```python
from build123d import *

# Parameters (mm, degrees)
SKETCH1_W           = 50
SKETCH1_H           = 50
SKETCH1_R           = 3.57
SKETCH1_R_2         = 2.51
BOSS_EXTRUDE1_DEPTH = 6.35
SKETCH2_R           = 6
SKETCH2_R_2         = 5.05
CUT_EXTRUDE1_DEPTH  = 1.75
SKETCH3_W           = 5.25
SKETCH3_H           = 6.7
CUT_EXTRUDE2_DEPTH  = 7
SKETCH4_W           = 2.785
SKETCH4_H           = 4.18
SKETCH4_W_2         = 2.79
SKETCH4_H_2         = 4.8
BOSS_EXTRUDE3_DEPTH = 6.7
FILLET1_R           = 6.17


with BuildPart() as part:
    # Sketch1 → Boss-Extrude1 (new body)
    with BuildSketch(Plane.XY):
        Rectangle(SKETCH1_W, SKETCH1_H)
        with Locations((-15, 15)):
            Circle(SKETCH1_R, mode=Mode.SUBTRACT)
        with Locations((15, 15)):
            Circle(SKETCH1_R, mode=Mode.SUBTRACT)
        with Locations((15, -15)):
            Circle(SKETCH1_R_2, mode=Mode.SUBTRACT)
        with Locations((-15, -15)):
            Circle(SKETCH1_R_2, mode=Mode.SUBTRACT)
        with Locations((-10, 0)):
            Circle(SKETCH1_R_2, mode=Mode.SUBTRACT)
        with Locations((0, 10)):
            Circle(SKETCH1_R_2, mode=Mode.SUBTRACT)
        with Locations((10, 0)):
            Circle(SKETCH1_R_2, mode=Mode.SUBTRACT)
        with Locations((0, -10)):
            Circle(SKETCH1_R_2, mode=Mode.SUBTRACT)
        Circle(SKETCH1_R_2, mode=Mode.SUBTRACT)
    extrude(amount=BOSS_EXTRUDE1_DEPTH)

    # Sketch2 → Cut-Extrude1 (cut)
    with BuildSketch(Plane.XY.offset(6.35)):
        with Locations((-15, 15)):
            Circle(SKETCH2_R)
        with Locations((15, 15)):
            Circle(SKETCH2_R)
        with Locations((-15, -15)):
            Circle(SKETCH2_R_2)
        with Locations((15, -15)):
            Circle(SKETCH2_R_2)
    extrude(amount=-CUT_EXTRUDE1_DEPTH, mode=Mode.SUBTRACT)

    # Sketch3 → Cut-Extrude2 (cut)
    with BuildSketch(Plane.XY.offset(6.35)):
        with Locations((-22.375, 0)):
            Rectangle(SKETCH3_W, SKETCH3_H)
        with Locations((22.375, 0)):
            Rectangle(SKETCH3_W, SKETCH3_H)
    extrude(amount=-CUT_EXTRUDE2_DEPTH, mode=Mode.SUBTRACT)

    # Sketch4 → Boss-Extrude3 (add)
    with BuildSketch(Plane.XZ.offset(-3.35)):
        with Locations((-23.6075, 2.09)):
            Rectangle(SKETCH4_W, SKETCH4_H)
        with Locations((23.605, 2.4)):
            Rectangle(SKETCH4_W_2, SKETCH4_H_2)
    extrude(amount=BOSS_EXTRUDE3_DEPTH)

    # Fillet1
    fillet1_edges = [part.edges().sort_by_distance(p)[0] for p in [
        (25, -25, 3.175),
        (-25, -25, 3.175),
        (-25, 25, 3.175),
        (25, 25, 3.175),
    ]]
    fillet(fillet1_edges, radius=FILLET1_R)


solid = part.part
```
Check sheet for the modelled part. Datum: model origin and axes. Units: mm. A direction names the side the tool comes from. Round coordinates to 2 decimals unless told otherwise and drop trailing zeros. Order: outer loops, then holes, each group sorted by start corner. A loop starts at its lowest first (then second) coordinate and runs counter-clockwise, first axis right, second up. Notation, with made-up numbers: (77.5, -13.75) -> (111.5, -13.75) arc R18 ccw to (111.5, 20.25) -> close; hole circle Ø7 at (-21, 71.25). An arc over 180 degrees is marked (long way). Use CSV: the item, a comma, the result in double quotes.
(1) Cross-section at D-D (z = 2). Count the separate pieces of the cut face and the enclosed holes in it, and give its area (3 significant figures).
Worked out:
separate pieces,"1"
enclosed holes,"11"
area,"2,220 mm²"
(2) Cross-section at C-C (y = -15). Record the boundary of the cut face in (x, z).
Worked out:
outline,"(-25, 0) -> (-17.51, 0) -> (-17.51, 4.6) -> (-20.05, 4.6) -> (-20.05, 6.35) -> (-25, 6.35) -> close; (-12.49, 0) -> (12.49, 0) -> (12.49, 4.6) -> (9.95, 4.6) -> (9.95, 6.35) -> (-9.95, 6.35) -> (-9.95, 4.6) -> (-12.49, 4.6) -> close; (17.51, 0) -> (25, 0) -> (25, 6.35) -> (20.05, 6.35) -> (20.05, 4.6) -> (17.51, 4.6) -> close"
(3) Tool access check on faces 1 (the face through (17, -17, 4.6)), 2 (the face through (0, 25, 3)), 3 (the face through (-22.215, 0, 2)), 4 (the face through (24, 0, 4.8)). Record the directions out of +Z, -Z, +X, -X, +Y, -Y that give a thin tool (end or side, any length) a straight path to the whole face; none if there is none.
Worked out:
face 1,"+Z"
face 2,"+Z, -Z, +X, -X, +Y"
face 3,"+Z, -Z"
face 4,"+Z, +X"
(4) Draft check along X on faces 5 (the face through (0, -5, 6.35)), 6 (the face through (-25, 0, 3)), 7 (the face through (-0.33, -7.51, 3.13)). Enter one of: pulls with the +X half, pulls with the -X half, needs draft (parallel to the pull), parting line crosses it, or undercut.
Worked out:
face 5,"needs draft"
face 6,"pulls with the -X half"
face 7,"undercut"
(5) Material ranges on line 1 along Y through (x, z) = (0, 3.5); line 2 along Y through (x, z) = (-15, 5); line 3 along X through (y, z) = (15, 1.1), recorded low to high. Write a range as from..to.
Worked out:
line 1,"-25..-12.51, -7.49..-2.51, 2.51..7.49, 12.51..25"
line 2,"-25..-20.05, -9.95..9, 21..25"
line 3,"-25..-18.57, -11.43..11.43, 18.57..25"
(6) Depth check by flat-ended pin: pin 1 (6 mm diameter, centred on x = 18, y = 17.5, fed in from +Z); pin 2 (1.4 mm diameter, centred on x = -24, y = 1.5, fed in from +Z); pin 3 (3 mm diameter, centred on x = -13.5, y = -13, fed in from +Z). Enter the tip coordinate at first touch or a pass-through.
Worked out:
pin 1,"z = 6.35"
pin 2,"z = 4.18"
pin 3,"z = 4.6"
(7) Cross-section at A-A (x = 0). Record the boundary of the cut face in (y, z).
Worked out:
outline,"(-25, 0) -> (-12.51, 0) -> (-12.51, 6.35) -> (-25, 6.35) -> close; (-7.49, 0) -> (-2.51, 0) -> (-2.51, 6.35) -> (-7.49, 6.35) -> close; (2.51, 0) -> (7.49, 0) -> (7.49, 6.35) -> (2.51, 6.35) -> close; (12.51, 0) -> (25, 0) -> (25, 6.35) -> (12.51, 6.35) -> close"
(8) Cross-section at B-B (x = -15). Record the boundary of the cut face in (y, z).
Worked out:
outline,"(-25, 0) -> (-17.51, 0) -> (-17.51, 4.6) -> (-20.05, 4.6) -> (-20.05, 6.35) -> (-25, 6.35) -> close; (-12.49, 0) -> (11.43, 0) -> (11.43, 4.6) -> (9, 4.6) -> (9, 6.35) -> (-9.95, 6.35) -> (-9.95, 4.6) -> (-12.49, 4.6) -> close; (18.57, 0) -> (25, 0) -> (25, 6.35) -> (21, 6.35) -> (21, 4.6) -> (18.57, 4.6) -> close"
